The listing builds one solid part. Answer for the finished solid, in the listing's coordinates (mm). A direction names the side the tool comes from. Give positions to 0.01 mm unless a question says otherwise; leave off trailing zeros. Order: outer loops, then holes, each group sorted by start corner. A loop starts at its lowest first (then second) coordinate and runs counter-clockwise, first axis right, second up.
Autodesk Inventor part; units mm, degrees
ref_plane "YZ Plane" through (0, 0, 0) normal (1, 0, 0) x (0, 1, 0)
ref_plane "XZ Plane" through (0, 0, 0) normal (0, 1, 0) x (-1, 0, 0)
ref_plane "XY Plane" through (0, 0, 0) normal (0, 0, 1) x (1, 0, 0)
sketch "Boceto1" plane through (0, 0, 0) normal (0, 1, 0) x (-1, 0, 0)
  circle A0 centre (0, 0) radius 3.15
  line L0 (6.889, 15) -> (3.889, 15)
  line L1 (3.889, -15) -> (6.889, -15)
  line L2 (6.889, -15) -> (6.889, 15)
  line L3 (0, 0) -> (3.15, 0) construction
  arc A1 (0.2346, 6.885) -> (0.2346, -6.885) centre (0, 0) ccw
  line L4 (3.889, 15) -> (3.889, 10.4169)
  line L5 (3.889, -15) -> (3.889, -10.4169)
  arc A2 (0.2346, 6.885) -> (3.889, 10.4169) centre (0.355, 10.4169) ccw
  arc A3 (3.889, -10.4169) -> (0.2346, -6.885) centre (0.355, -10.4169) ccw
  line L6 (2.9445, 5.1) -> (5.889, 0) construction
  line L7 (5.889, 0) -> (2.9445, -5.1) construction
  line L8 (2.9445, -5.1) -> (-2.9445, -5.1) construction
  line L9 (-2.9445, -5.1) -> (-5.889, 0) construction
  line L10 (-5.889, 0) -> (-2.9445, 5.1) construction
  line L11 (-2.9445, 5.1) -> (2.9445, 5.1) construction
  line L12 (5.889, 0) -> (6.889, 0) construction
  line L13 (-5.889, 0) -> (-6.889, 0) construction
  dimension "d0" = 6.3
  dimension "d3" = 10.2
  dimension "d4" = 1
  dimension "d5" = 3
  dimension "d12" = 30
extrude "Extrusión1" add sketch "Boceto1" along normal blind 57
sketch "Boceto2" plane through (0, 0, 0) normal (0, -1, 0) x (1, 0, 0)
  line L0 (-5.7735, 0) -> (-2.8868, 5)
  line L1 (-2.8868, 5) -> (2.8868, 5)
  line L2 (2.8868, 5) -> (5.7735, 0)
  line L3 (5.7735, 0) -> (2.8868, -5)
  line L4 (2.8868, -5) -> (-2.8868, -5)
  line L5 (-2.8868, -5) -> (-5.7735, 0)
  point P0 (0, 0)
  point P1 (0, 0)
  dimension "d8" = 10
extrude "Extrusión2" cut sketch "Boceto2" against normal blind 6
sketch "Boceto4" plane through (-6.889, 0, -15) normal (-1, 0, 0) x (0, 0, 1)
  line L0 (0, 0) -> (0, 57)
  line L1 (0, 28.5) -> (30, 28.5) construction
  line L2 (30, 0) -> (30, 57)
  line L3 (0, 36) -> (2, 36)
  line L4 (2, 36) -> (2, 40)
  line L5 (2, 40) -> (0, 40)
  line L6 (0, 40) -> (0, 36)
  line L7 (30, 36) -> (28.1744, 36)
  line L8 (28.1744, 36) -> (28.1744, 40)
  line L9 (28.1744, 40) -> (30, 40)
  line L10 (30, 40) -> (30, 36)
  line L11 (0, 21) -> (2, 21)
  line L12 (2, 21) -> (2, 17)
  line L13 (2, 17) -> (0, 17)
  line L14 (0, 17) -> (0, 21)
  line L15 (30, 21) -> (28.1744, 21)
  line L16 (28.1744, 21) -> (28.1744, 17)
  line L17 (28.1744, 17) -> (30, 17)
  line L18 (30, 17) -> (30, 21)
  line L19 (2, 40) -> (28.1744, 40) construction
  line L20 (2, 36) -> (28.1744, 36) construction
  line L21 (2, 21) -> (28.1744, 21) construction
  line L22 (2, 17) -> (28.1744, 17) construction
  point P0 (15, 0)
  dimension "d13" = 2
  dimension "d14" = 4
  dimension "d15" = 15
extrude "Extrusión3" cut sketch "Boceto4" against normal up to next
fillet "Empalme1" radius 5 4 edges at (-5.389, 57, -15) (-5.389, 57, 15) (-5.389, 0, 15) (-5.389, 0, -15)
properties part number "Soporte ESC"
1) Straight lines are drawn through the part: probe 1 along Z at (x, y) = (0.25, 38); probe 2 along X at (y, z) = (43, 0); probe 3 along X at (y, z) = (10.5, 12.5). For each, find the intervals that lie inside material, in ascending order.
Geometry says:
probe 1: z = -6.88 to -3.14, 3.14 to 6.88
probe 2: x = -6.89 to -3.15, 3.15 to 6.89
probe 3: x = -6.89 to -3.89
2) Find section D-D (z = -7.5). Write down the section's boundary in (x, y), then the cut area to 3 significant figures.
Geometry says:
outline: (-6.89, 0) - (-2.35, 0) - (-2.35, 57) - (-6.89, 57) - close
area: 259 mm2
3) Find section B-B (z = 11). Write down the section's boundary in (x, y), then the cut area to 3 significant figures.
Geometry says:
outline: (-6.89, 0.1) - (-3.89, 0.1) - (-3.89, 56.9) - (-6.89, 56.9) - close
area: 170 mm2
4) Find section A-A (y = 4). Write down the section's boundary in (x, z) (1 decimal).
Geometry says:
outline: (-6.9, -14.9) - (-3.9, -14.9) - (-3.9, -10.4) arc R3.5 cw to (-0.2, -6.9) arc R6.9 ccw (long way) to (-0.2, 6.9) arc R3.5 cw to (-3.9, 10.4) - (-3.9, 14.9) - (-6.9, 14.9) - close; hole (-5.8, 0) - (-2.9, -5) - (2.9, -5) - (5.8, 0) - (2.9, 5) - (-2.9, 5) - close
5) Given P1, Ø2, axis at x = -5, z = 13.5, coming from the -Y side; P2, Ø1.5, axis at x = -5.5, z = 14.5, coming from the -Y side; P3, Ø5, axis at y = 37.5, z = -12.5, coming from the +X side, each flat-ended and moving along its own axis, determine where each tip first touches the part or whether it passes through.
Geometry says:
P1: stops at y = 0.67
P2: stops at y = 1.69
P3: stops at x = -3.86
6) Find section C-C (y = 28.5). Write down the section's boundary in (x, z) (3 decimals).
Geometry says:
outline: (-6.889, -15) - (-3.889, -15) - (-3.889, -10.417) arc R3.534 cw to (-0.235, -6.885) arc R6.889 ccw (long way) to (-0.235, 6.885) arc R3.534 cw to (-3.889, 10.417) - (-3.889, 15) - (-6.889, 15) - close; hole circle Ø6.3 at (0, 0)
7) For a pull along X with two mould halves and no side action, classify faces 5 (the flat face through (-4.31, 2.958, -2.535)), 6 (the flat face through (-5, 38, 13.174)), 7 (the flat face through (-6.889, 28, 0)) as +X half, -X half, draft (parallel to the pull), parting line (faces both ways), or undercut.
Geometry says:
face 5: undercut
face 6: draft
face 7: -X half
8) A tool of negligible diameter and unlimited length cuts with its end or side. For faces 1 (the flat face through (-5, 21, -14)), 2 (the flat face through (-5, 17, 14)), 3 (the flat face through (4.31, 2.958, 2.535)), 4 (the cylindrical face through (-5, 56, -13)), from which of +Z, -Z, +X, -X, +Y, -Y can it reach the whole face along a straight path? Write none if from no direction.
Geometry says:
face 1: -Z, +X, -X
face 2: +Z, +X, -X
face 3: -Y
face 4: -Z, +X, -X, +Y
